Geometry: see drawing. Coordinates: mm, zero at the bounding-box minimum. A direction names the side the tool comes from. Coordinates: 2 decimals unless noted, no trailing zeros. Write each loop counter-clockwise with the first axis right and the second up, starting at its lowest first coordinate (ties: lowest second). Pieces come first, ordered by that corner, then holes. Notation, with made-up numbers: M 85,15.5 L 123,15.5 A22 cw 123,38.5 Z; hole C -27,78.5 d2. An arc over 180 degrees is marked long. Answer as CSV lines item,"result". Start each with the question number.
1. Section B-B on z = 4.5. Return the cut outline in (x, y), plus the area to 3 significant figures.
2. Mould query, pull axis X, two halves, no side actions, for the marked faces 1, 2 and 3. Classes: pulls with the +X half, pulls with the -X half, needs draft (parallel to the pull), parting line crosses it, or undercut.
3. Contact query for flat-ended pins moving along their axis: pin 1 Ø3 at (x, z) = (2, 4) entering from -Y; pin 2 Ø3 at (x, y) = (5.5, 8.5) entering from +Z; pin 3 Ø1.5 at (x, z) = (7.5, 2.5) entering from +Y. Output: stop coordinate, or through.
4. Section A-A on y = 5. Return the cut outline in (x, z) (1 decimal), plus the area to 3 significant figures.
5. Section D-D on z = 1.5. Return the cut outline in (x, y).
6. Line query: probe 1 along Y at (x, z) = (5, 4.2); probe 2 along Z at (x, y) = (0.5, 5.75); probe 3 along Z at (x, y) = (3.75, 5.25). Output: solid intervals per line, ascending. Write a range as [from, to].
7. Reachability of the marked faces 4 and 5 from +Z, -Z, +X, -X, +Y, -Y: full face, straight path, thin tool, end or side. Return the list, or none.
8. Section C-C on x = 2. Return the cut outline in (y, z), plus the area to 3 significant figures.
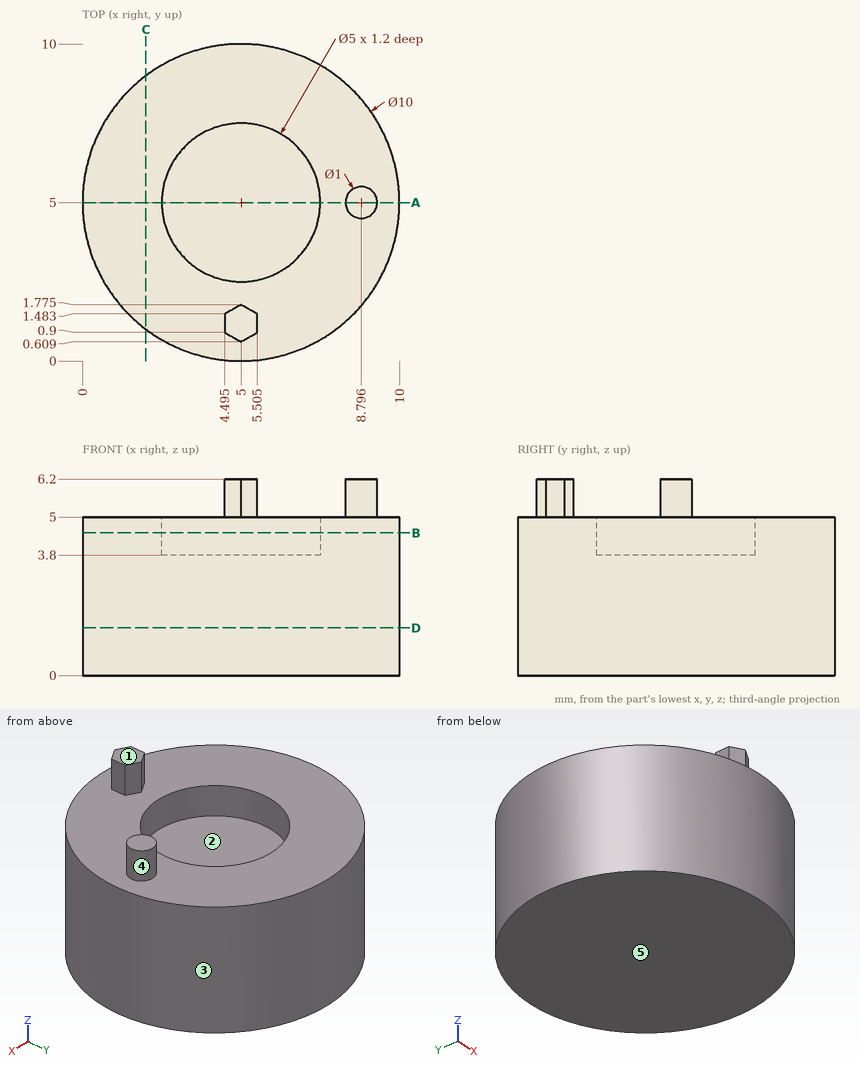
Values:
1,outline,"C 5,5 d10; hole C 5,5 d5"
1,area,"58.9 mm²"
2,face 1,"needs draft"
2,face 2,"undercut"
2,face 3,"parting line crosses it"
3,pin 1,"y = 0.23"
3,pin 2,"z = 5"
3,pin 3,"y = 9.68"
4,outline,"M 0,0 L 10,0 L 10,5 L 9.3,5 L 9.3,6.2 L 8.3,6.2 L 8.3,5 L 7.5,5 L 7.5,3.8 L 2.5,3.8 L 2.5,5 L 0,5 Z"
4,area,"45.2 mm²"
5,outline,"C 5,5 d10"
6,probe 1,"[0, 2.5], [7.5, 10]"
6,probe 2,"[0, 5]"
6,probe 3,"[0, 3.8]"
7,face 4,"+Z"
7,face 5,"-Z, +X, -X, +Y, -Y"
8,outline,"M 1,0 L 9,0 L 9,5 L 1,5 Z"
8,area,"40.0 mm²"
